Autodesk Inventor part; units mm, degrees
ref_plane "YZ Plane" through (0, 0, 0) normal (1, 0, 0) x (0, 1, 0)
ref_plane "XZ Plane" through (0, 0, 0) normal (0, 1, 0) x (-1, 0, 0)
ref_plane "XY Plane" through (0, 0, 0) normal (0, 0, 1) x (1, 0, 0)
sketch "Szkic1" plane through (0, 0, 0) normal (0, 1, 0) x (-1, 0, 0)
  line L0 (-26, 80) -> (26, 80)
  line L1 (26, 80) -> (26, -80)
  line L2 (26, -80) -> (-26, -80)
  line L3 (-26, -80) -> (-26, 80)
  line L4 (-26, 80) -> (26, -80) construction
  line L5 (26, 80) -> (-26, -80) construction
  point P0 (0, 0)
  dimension "d0" = 52
  dimension "d1" = 160
extrude "Wyciągnięcie proste1" add sketch "Szkic1" along normal blind 30
shell "Skorupa1" thickness 3.5 removed faces 1 at (8.6667, 30, 26.6667)
sketch "Szkic3" plane through (-26, 0, 80) normal (0, 0, 1) x (1, 0, 0)
  line L0 (52, 0) -> (52, 30)
  line L1 (0, 0) -> (52, 0)
  line L2 (52, 0) -> (52, 30)
  line L3 (52, 30) -> (0, 30)
  line L4 (0, 30) -> (0, 0)
  line L5 (52, 0) -> (0, 0)
  line L6 (52, 30) -> (0, 30)
  line L7 (48.5, 0) -> (3.5, 0)
  line L8 (3.5, 0) -> (3.5, 30)
  line L9 (3.5, 30) -> (48.5, 30)
  line L10 (48.5, 30) -> (48.5, 0)
  line L11 (3.5, 25) -> (48.5, 25)
  line L12 (48.5, 25) -> (48.5, 5)
  line L13 (48.5, 5) -> (3.5, 5)
  line L14 (3.5, 5) -> (3.5, 25)
  circle A0 centre (13, 15) radius 8
  circle A1 centre (39, 15) radius 8
  point P0 (26, 0)
  point P1 (3.5, 15)
  dimension "d7" = 52
  dimension "d8" = 30
  dimension "d9" = 3.5
  dimension "d10" = 3.5
  dimension "d11" = 45
  dimension "d12" = 45
  dimension "d13" = 20
  dimension "d14" = 5
  dimension "d15" = 16
  dimension "d16" = 16
  dimension "d17" = 26
  dimension "d18" = 10
  dimension "d19" = 9.5
extrude "Wyciągnięcie proste2" cut sketch "Szkic3" against normal up to next contours A0 | A1
sketch "Szkic4" plane through (-26, 0, 80) normal (0, 0, 1) x (1, 0, 0)
  line L0 (0, 0) -> (0, 30)
  line L1 (0, 30) -> (52, 30)
  line L2 (0, 0) -> (52, 0)
  line L3 (52, 0) -> (52, 30)
  line L4 (52, 30) -> (0, 30)
  line L5 (0, 30) -> (0, 0)
  circle A0 centre (13, 15) radius 8
  circle A1 centre (13, 15) radius 8
  circle A2 centre (39, 15) radius 8
  circle A3 centre (39, 15) radius 8
  point P0 (26, 0)
  point P1 (47, 22.5)
extrude "Wyciągnięcie proste3" add sketch "Szkic4" along normal blind 4
sketch "Szkic8" plane through (0, 0, 0) normal (0, -1, 0) x (1, 0, 0)
  line L0 (26, 10) -> (22, 10)
  line L1 (22, 10) -> (22, -10)
  line L2 (22, -10) -> (26, -10)
  line L3 (26, -10) -> (26, 10)
  line L4 (26, -80) -> (26, 84)
  point P0 (0, 0)
  point P1 (26, 0)
  point P2 (26, 2)
  dimension "d46" = 20
  dimension "d47" = 4
extrude "Wyciągnięcie proste6" add sketch "Szkic8" along normal blind 20
sketch "Szkic11" plane through (0, 0, 0) normal (0, -1, 0) x (1, 0, 0)
  line L0 (-26, -80) -> (-26, 84)
  line L1 (-26, 15) -> (-22, 15)
  line L2 (-22, 15) -> (-22, -15)
  line L3 (-22, -15) -> (-26, -15)
  line L4 (-26, -15) -> (-26, 15)
  point P0 (0, 0)
  dimension "d55" = 4
  dimension "d56" = 30
  dimension "d57" = 15
extrude "Wyciągnięcie proste8" add sketch "Szkic11" along normal blind 20
sketch "Szkic12" plane through (-26, 0, -80) normal (-1, 0, 0) x (0, 0, 1)
  circle A0 centre (80, -10) radius 5
  line L0 (95, 0) -> (95, -20)
  line L1 (95, -20) -> (65, -20)
  point P0 (80, 0)
  dimension "d60" = 10
  dimension "d61" = 15
  dimension "d62" = 10
extrude "Wyciągnięcie proste9" cut sketch "Szkic12" against normal blind 20
sketch "Szkic13" plane through (-26, 0, -80) normal (-1, 0, 0) x (0, 0, 1)
  line L0 (95, -20) -> (65, -20)
  line L1 (95, -20) -> (109.2717, -5.7283)
  line L2 (95, -20) -> (115.1833, -20) construction
  line L3 (109.2717, -5.7283) -> (115, 0)
  line L4 (95, 0) -> (164, 0)
  line L5 (95, 0) -> (95, -20)
  line L6 (95, 0) -> (95, -20)
  line L7 (65, 0) -> (65, -20)
  line L8 (65, -20) -> (48.9371, -3.9371)
  line L9 (65, -20) -> (87.7163, -20) construction
  line L10 (48.9371, -3.9371) -> (45, 0)
  line L11 (0, 0) -> (70, 0)
  line L12 (95, 0) -> (65, 0)
  line L13 (65, 0) -> (65, -20)
  line L14 (65, 0) -> (45, 0)
  line L15 (115, 0) -> (95, 0)
  point P0 (80, 0)
  dimension "d65" = 45
  dimension "d67" = 135
extrude "Wyciągnięcie proste10" add sketch "Szkic13" against normal blind 4 contours L5 L4 L3 L1 | L8 L10 L11 L7
sketch "Szkic14" plane through (26, 0, -80) normal (1, 0, 0) x (0, 0, -1)
  line L0 (-70, -20) -> (-50, 0)
  line L1 (-70, -20) -> (-41.7157, -20) construction
  line L2 (-70, 0) -> (-70, -20)
  line L3 (-50, 0) -> (-70, 0)
  line L4 (-70, 0) -> (-70, -20)
  line L5 (-90, 0) -> (-90, -20)
  line L6 (-90, -20) -> (-110, 0)
  line L7 (-90, -20) -> (-61.7157, -20) construction
  line L8 (-110, 0) -> (-90, 0)
  line L9 (-90, 0) -> (-90, -20)
  point P0 (-80, 0)
  point P1 (-115, 0)
  point P2 (-45, 0)
  dimension "d70" = 45
  dimension "d71" = 135
extrude "Wyciągnięcie proste11" add sketch "Szkic14" against normal blind 4
sketch "Szkic15" plane through (22.5, 3.5, 76.5) normal (0, 0, -1) x (-1, 0, 0)
  line L0 (0, 26.5) -> (45, 26.5)
  line L1 (45, 26.5) -> (0, 26.5)
  line L2 (0, 26.5) -> (0, -1)
  line L3 (0, -1) -> (45, -1)
  line L4 (45, -1) -> (45, 26.5)
  point P0 (22.5, -3.5)
  point P1 (0, 26.5)
  dimension "d74" = 27.5
extrude "Wyciągnięcie proste12" cut sketch "Szkic15" against normal blind 4
sketch "Szkic17" plane through (-22.5, 3.5, -76.5) normal (1, 0, 0) x (0, 0, -1)
  line L0 (0, 26.5) -> (-4.1115, 3.1827)
  line L1 (0, 26.5) -> (23.677, 26.5) construction
  line L2 (-4.1115, 3.1827) -> (-5.1108, -2.485)
  line L3 (-4.6727, 0) -> (0, 0)
  line L4 (-157, 26.5) -> (0, 26.5)
  line L5 (0, 0) -> (0, 26.5)
  point P0 (-76.5, -3.5)
  dimension "d77" = 100
extrude "Wyciągnięcie proste13" add sketch "Szkic17" along normal blind 48
sketch "Szkic20" plane through (22.5, 3.5, 76.5) normal (0, 0, 1) x (1, 0, 0)
  line L0 (0, -1) -> (0, 26.5)
  line L1 (-45, 0) -> (0, 0)
  line L2 (0, 0) -> (0, -1)
  line L3 (0, -1) -> (-45, -1)
  line L4 (-45, -1) -> (-45, 0)
  point P0 (-22.5, -3.5)
extrude "Wyciągnięcie proste14" add sketch "Szkic20" along normal blind 7
sketch "Szkic25" plane through (26, 0, -80) normal (1, 0, 0) x (0, 0, -1)
  circle A0 centre (-80, -10) radius 5
  circle A1 centre (-80, -10) radius 1.25
  point P0 (-80, 0)
  dimension "d84" = 2.5
extrude "Wyciągnięcie proste15" cut sketch "Szkic25" against normal up to next contours A1
equation "\"d10\" = d9"
equation "\"d14\" = -0.5 * d13 + 0.5 * d8"
equation "\"d18\" = 0.5 * d13"
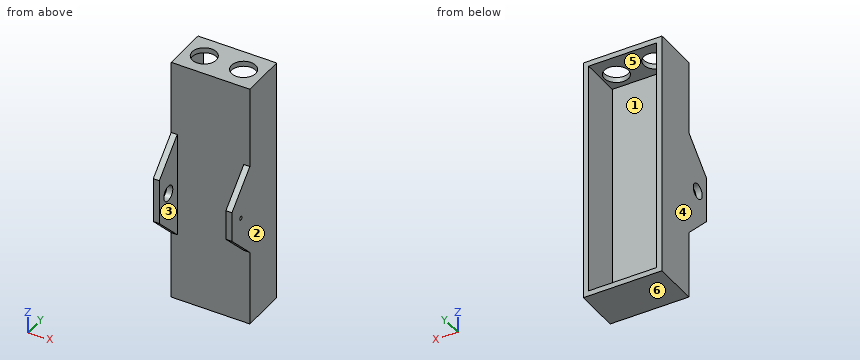
Can you work these out from the model? Positions are in its coordinate system, mm. Face numbers are marked on the shaded views. A direction names the side the tool comes from. Round coordinates to 2 decimals unless told otherwise and drop trailing zeros. Write each loop counter-clockwise with the first axis right and the second up, starting at its lowest first coordinate (ties: lowest second). Pieces come first, ordered by that corner, then holes. Notation, with made-up numbers: (78.25, -13.5) -> (83.25, -13.5) arc R21 cw to (83.25, 16.5) -> close; hole circle Ø2 at (-38.5, 78). An arc over 180 degrees is marked (long way). Use one line per item in the form item = value. Start each with the question number.
Q1. Imagine slicing it at A-A (x = -13). Please give me the cut outline in (y, z).
Q2. We'd pull the mould along X, two halves only. Please class the marked faces 4, 5 and 6: +X half, -X half, draft (parallel to the pull), parting line (faces both ways), or undercut.
Q3. Imagine slicing it at B-B (y = 21). Please give me the cut outline in (x, z).
Q4. Imagine slicing it at C-C (x = 0). Please give me the cut outline in (y, z), then the cut area to 3 significant figures.
Q5. Imagine slicing it at D-D (z = -49). Please give me the cut outline in (x, y), then the cut area to 4 significant figures.
Q6. Which directions (+Z, -Z, +X, -X, +Y, -Y) give clear straight access to the entire face, cutting with the end or side of a thin tool? Please do the marked faces 1, 2 and 3.
Q7. I'm going to push flat-ended pins straight in: P1, Ø12, axis at x = 14, y = -8, coming from the +Z side; P2, Ø13, axis at x = 13, y = 15, coming from the +Z side; P3, Ø12, axis at x = 5, z = -40.5, coming from the +Y side; P4, Ø10, axis at x = 16, z = 47.5, coming from the -Y side. Where does each tip first touch, or does it pass through?
Q8. If I drill on probe 1 along Y at (x, z) = (-13, 82.85); probe 2 along X at (y, z) = (19.5, -34); probe 3 along Y at (x, z) = (23.8, 0), over which ranges is the centre line in solid material (lowest first)? Write a range as [from, to].
Worked out:
q1.outline = (0, -80) -> (30, -80) -> (30, -76.5) -> (6.68, -72.39) -> (3.5, -71.83) -> (3.5, 80.5) -> (7, 80.5) -> (7, 84) -> (0, 84) -> close; (23, 80.5) -> (30, 80.5) -> (30, 84) -> (23, 84) -> close
q2.face_4 = -X half
q2.face_5 = undercut
q2.face_6 = draft
q3.outline = (-26, -80) -> (26, -80) -> (26, 84) -> (18.29, 84) -> (18.29, 80.5) -> (22.5, 80.5) -> (22.5, -74.91) -> (-22.5, -74.91) -> (-22.5, 80.5) -> (-18.29, 80.5) -> (-18.29, 84) -> (-26, 84) -> close; (-7.71, 80.5) -> (7.71, 80.5) -> (7.71, 84) -> (-7.71, 84) -> close
q4.outline = (0, -80) -> (30, -80) -> (30, -76.5) -> (6.68, -72.39) -> (3.5, -71.83) -> (3.5, 80.5) -> (30, 80.5) -> (30, 84) -> (0, 84) -> close
q4.area = 821 mm^2
q5.outline = (-26, 0) -> (26, 0) -> (26, 30) -> (22.5, 30) -> (22.5, 3.5) -> (-22.5, 3.5) -> (-22.5, 30) -> (-26, 30) -> close
q5.area = 367.5 mm^2
q6.face_1 = +Y
q6.face_2 = +Z, -Z, +X, +Y, -Y
q6.face_3 = +Z, -Z, -Y
q7.P1 = through
q7.P2 = -72.71
q7.P3 = 3.5
q7.P4 = 0
q8.probe_1 = [0, 7], [23, 30]
q8.probe_2 = [-26, -22.5], [22.5, 26]
q8.probe_3 = [-20, -11.25], [-8.75, 30]
